Could you check a few things on this drawing? It's one solid part, dimensions in mm from its lowest x, y, z. A direction names the side the tool comes from. Give positions to 0.01 mm unless a question says otherwise; leave off trailing zeros. Loops run counter-clockwise (first coordinate to the right, second up) from the corner with the lowest first, then second, coordinate; pieces in that order, holes last. Notation, with made-up numbers: (26, -16.75) - (60, -16.75) arc R9 ccw to (60, -12.75) - close; hole circle Ø1 at (-25, 18.25). An arc over 180 degrees is marked (long way). Use a Markdown table: item, result.
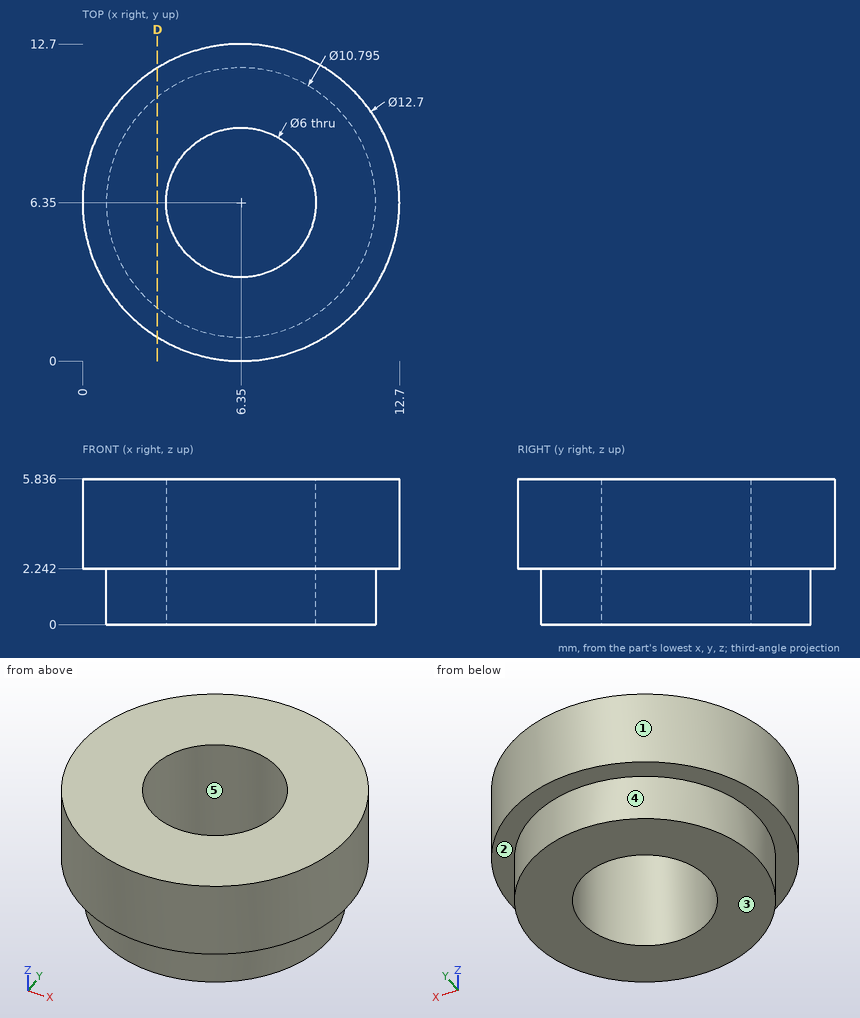
(1) If I drill on line 1 (Y direction, x = 6.35, z = 1.75); line 2 (Y direction, x = 6.35, z = 3.9); line 3 (X direction, y = 8, z = 3.8) (1 decimal), over which ranges is the centre line in solid material (lowest first)?
A:
| item | result |
|---|---|
| line 1 | 0.95 to 3.35, 9.35 to 11.75 |
| line 2 | 0 to 3.35, 9.35 to 12.7 |
| line 3 | 0.2 to 3.8, 8.9 to 12.5 |
(2) On a 3-axis mill with a long thin cutter (end or side, diameter ignored), from which of +Z, -Z, +X, -X, +Y, -Y can I reach the whole of each face in a straight line? I mean the marked faces 1 and 2. Say none if no direction works.
A:
| item | result |
|---|---|
| face 1 | +Z, -Z |
| face 2 | -Z |
(3) We'd pull the mould along Y, two halves only. Please class the marked faces 3, 4 and 5: pulls with the +Y half, pulls with the -Y half, needs draft (parallel to the pull), parting line crosses it, or undercut.
A:
| item | result |
|---|---|
| face 3 | needs draft |
| face 4 | parting line crosses it |
| face 5 | undercut |
(4) Will these pins go through, and if not, where does the flat tip stop? pin 1 (1 mm diameter, centred on y = 8, z = 3, fed in from +X) (1 decimal); pin 2 (1.5 mm diameter, centred on x = 5, z = 4.5, fed in from +Y); pin 3 (1 mm diameter, centred on y = 5.5, z = 1, fed in from -X).
A:
| item | result |
|---|---|
| pin 1 | x = 12.6 |
| pin 2 | y = 12.67 |
| pin 3 | x = 0.96 |
(5) Suppose I cut it at D-D on x = 3. Write out the boundary of the cut face in (y, z) (1 decimal).
A:
| item | result |
|---|---|
| outline | (1, 2.2) - (2.1, 2.2) - (2.1, 0) - (10.6, 0) - (10.6, 2.2) - (11.7, 2.2) - (11.7, 5.8) - (1, 5.8) - close |
